from build123d import *

# Parameters (mm, degrees)
SKETCH2_W               = 215.9
SKETCH2_H               = 10.7188
BOSS_EXTRUDE1_DEPTH     = 4.7498
CUT_EXTRUDE1_DEPTH      = 127
CUT_EXTRUDE2_DEPTH      = 184.509479274
CUT_EXTRUDE2_DEPTH_BACK = 184.509479274


with BuildPart() as part:
    # Sketch2 → Boss-Extrude1 (new body)
    with BuildSketch(Plane(origin=(0, 0, 0), x_dir=(1, 0, 0), z_dir=(0, 1, 0))):
        Polygon((108.966, 101.612438876), (0, 0), (215.9, 0), (254, 0), (223.266, 101.612438876), align=None)
        with Locations((107.95, -5.3594)):
            Rectangle(SKETCH2_W, SKETCH2_H)
    extrude(amount=BOSS_EXTRUDE1_DEPTH)

    # Sketch11 → Cut-Extrude1 (cut)
    with BuildSketch(Plane(origin=(21.289272777, 0, 70.386377589), x_dir=(-0.9571749920693967, 0, 0.2895099904268422), z_dir=(-0.2895099904268422, 0, -0.9571749920693967))):
        Polygon((-243.122447986, 2.3749), (-235.083929839, 4.7498), (-235.083929839, 6.735693681), (-246.008613283, 6.735693681), (-246.008613283, -1.683735196), (-235.083929839, -1.683735196), (-235.083929839, 0), align=None)
    extrude(amount=CUT_EXTRUDE1_DEPTH, mode=Mode.SUBTRACT)

    # Sketch9 → Cut-Extrude2 (cut, two sides: drawn at the far end of the back side and taken through both)
    with BuildSketch(Plane(origin=(108.966, 0, -101.612438876), x_dir=(0.6819983600624973, 0, 0.7313537016191718), z_dir=(-0.7313537016191718, 0, 0.6819983600624973)).offset(-CUT_EXTRUDE2_DEPTH_BACK)):
        Polygon((0, 2.3749), (12.992733122, 0), (12.992733122, -1.975315997), (-2.377492565, -1.975315997), (-2.377492565, 7.448660166), (12.992733122, 7.448660166), (12.992733122, 4.7498), align=None)
    extrude(amount=CUT_EXTRUDE2_DEPTH + CUT_EXTRUDE2_DEPTH_BACK, mode=Mode.SUBTRACT)


solid = part.part
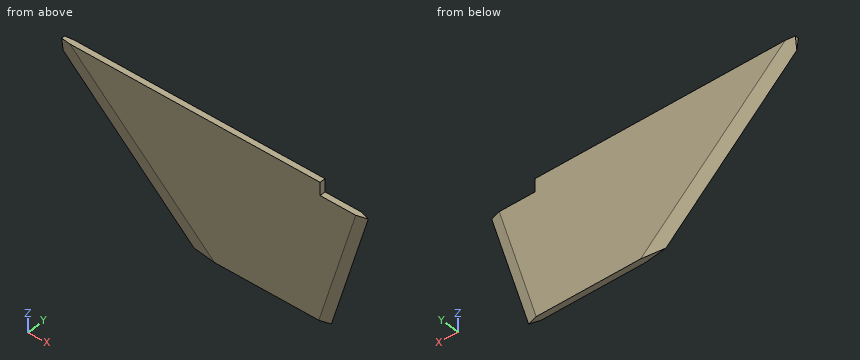
Verification items for the finished model (mm, model axes). Give positions to 0.01 mm unless a question says otherwise; leave off trailing zeros. Order: outer loops, then holes, each group sorted by start corner. A loop starts at its lowest first (then second) coordinate and runs counter-clockwise, first axis right, second up. Notation, with made-up numbers: M 49.5,33 L 71.5,33 A8 cw 71.5,40 Z; hole C -33,88 d1. An arc over 180 degrees is marked long. Use one line per item in the form item = value. Start each with the question number.
Q1. Go/stop test with flat-tipped pins: pin 1 Ø12 at (x, z) = (142, -70) entering from -Y; pin 2 Ø1.5 at (x, y) = (55, 3) entering from -Z. Record where each tip stops, or that it passes through.
Q2. Section check D-D (z = -90). Enter the section's corners in (x, y), then the cut area to 3 significant figures.
Q3. Section check A-A (x = 86). Enter the section's corners in (y, z), then the cut area to 3 significant figures.
Q4. Section check C-C (x = 231.5). Enter the section's corners in (y, z).
Q5. Section check B-B (z = -46.5). Enter the section's corners in (x, y), then the cut area to 3 significant figures.
Q6. Scan lines: line 1 along Y through (x, z) = (108.5, -97); line 2 along Y through (x, z) = (232.5, -53.5). Record each from-to range of solid material in increasing order. Write a range as [from, to].
Evaluation:
q1.pin_1 = 0
q1.pin_2 = -51.67
q2.outline = M 96.51,2.37 L 115.56,0 L 218.38,0 L 226.78,2.37 L 218.38,4.75 L 115.56,4.75 Z
q2.area = 554 mm2
q3.outline = M 0,-62.43 L 2.37,-80.2 L 4.75,-62.43 L 4.75,10.72 L 0,10.72 Z
q3.area = 390 mm2
q4.outline = M 0,-46.62 L 2.37,-74.39 L 4.75,-46.62 L 4.75,0 L 0,0 Z
q5.outline = M 49.87,2.37 L 68.92,0 L 231.54,0 L 239.94,2.37 L 231.54,4.75 L 68.92,4.75 Z
q5.area = 838 mm2
q6.line_1 = [1.82, 2.93]
q6.line_2 = [0.87, 3.88]
